from build123d import *

# Parameters (mm, degrees)
CROQUIS1_R               = 18.5
SALIENTE_EXTRUIR1_DEPTH  = 5
CROQUIS2_R               = 0.75
CORTAR_EXTRUIR1_DEPTH    = 5
CROQUIS3_R               = 17.5
CROQUIS3_R_2             = 2.5
CORTAR_EXTRUIR4_DEPTH    = 5
SALIENTE_EXTRUIR11_START = -5
CROQUIS6_W               = 17.427059278
CROQUIS6_H               = 4
SALIENTE_EXTRUIR11_DEPTH = 5
CROQUIS8_W               = 17.261171747
CROQUIS8_H               = 4
SALIENTE_EXTRUIR12_DEPTH = 5


with BuildPart() as part:
    # Croquis1 → Saliente-Extruir1 (new body)
    with BuildSketch(Plane.XY):
        with Locations((-21.322301086, 7.958835432)):
            Circle(CROQUIS1_R)
    extrude(amount=SALIENTE_EXTRUIR1_DEPTH)

    # Croquis2 → Cortar-Extruir1 (cut)
    with BuildSketch(Plane(origin=(0, 0, 0), x_dir=(-1, 0, 0), z_dir=(0, 0, -1))):
        with Locations((21.322301086, 7.958835432)):
            Circle(CROQUIS2_R)
    extrude(amount=-CORTAR_EXTRUIR1_DEPTH, mode=Mode.SUBTRACT)

    # Croquis3 → Cortar-Extruir4 (cut)
    with BuildSketch(Plane.XY.offset(5)):
        with Locations((-21.322301086, 7.958835432)):
            Circle(CROQUIS3_R)
        with Locations((-21.322301086, 7.958835432)):
            Circle(CROQUIS3_R_2, mode=Mode.SUBTRACT)
    extrude(amount=-CORTAR_EXTRUIR4_DEPTH, mode=Mode.SUBTRACT)


with BuildPart() as cortar_extruir4_piece_1:
    # of the separate pieces the step leaves, piece 1, a body of its own (cortar_extruir4_pieces)
    add(part.part.solids().sort_by_distance((-2.822301086, 7.958835432, 0))[0])



with BuildPart() as cortar_extruir4_piece_2:
    # of the separate pieces the step leaves, piece 2, a body of its own (cortar_extruir4_pieces)
    add(part.part.solids().sort_by_distance((-18.822301086, 7.958835432, 0))[0])


with BuildPart() as cortar_extruir4_piece_1_1:
    add(cortar_extruir4_piece_1.part)

    add(cortar_extruir4_piece_2.part)  # Saliente-Extruir11 merges Cortar-Extruir4 piece 2
    # Croquis6 → Saliente-Extruir11 (add)
    with BuildSketch(Plane.XY.offset(5).offset(SALIENTE_EXTRUIR11_START)):
        with Locations((-31.000345605, 7.958835432)):
            Rectangle(CROQUIS6_W, CROQUIS6_H)
    extrude(amount=SALIENTE_EXTRUIR11_DEPTH)

    # Croquis8 → Saliente-Extruir12 (add)
    with BuildSketch(Plane.XY.offset(5)):
        with Locations((-11.561312802, 7.958835432)):
            Rectangle(CROQUIS8_W, CROQUIS8_H)
    extrude(amount=-SALIENTE_EXTRUIR12_DEPTH)


solid = cortar_extruir4_piece_1_1.part
Here's how the part is built. I have some questions about the finished solid (model axes, mm). A direction names the side the tool comes from. Round coordinates to 2 decimals unless told otherwise and drop trailing zeros. Order: outer loops, then holes, each group sorted by start corner. A loop starts at its lowest first (then second) coordinate and runs counter-clockwise, first axis right, second up. Notation, with made-up numbers: M -4,35 L 17,35 A33 cw 17,68 Z; hole C 37,45.25 d7. An arc over 180 degrees is marked long. One line per question, with ' | ' between items.
1) I'm going to push flat-ended pins straight in: pin 1 Ø2.5 at (x, z) = (-27, 2.5) entering from -Y; pin 2 Ø1.5 at (x, z) = (-12, 3) entering from -Y; pin 3 Ø2.5 at (x, z) = (-14, 3) entering from +Y. Where does each tip first touch, or does it pass through?
Checked values:
pin 1: stops at y = -10 | pin 2: stops at y = -8.44 | pin 3: stops at y = 25.43
2) I need wall thicknesses on line 1 (Y direction, x = -31, z = 0.55); line 2 (Y direction, x = -13.5, z = 1.9); line 3 (X direction, y = 16.5, z = 2.1). Which ranges of each line are inside material? Lowest first, please.
Checked values:
line 1: y = -7.81 to -6.62, 5.96 to 9.96, 22.54 to 23.73 | line 2: y = -8.81 to -7.7, 5.96 to 9.96, 23.61 to 24.72 | line 3: x = -37.73 to -36.6, -6.05 to -4.91
3) Imagine slicing it at A-A, the plane y = 17.5. Write out the boundary of the cut face in (x, z), plus the area to 3 significant figures.
Checked values:
outline: M -37.17,0 L -35.99,0 L -35.99,5 L -37.17,5 Z; M -6.65,0 L -5.47,0 L -5.47,5 L -6.65,5 Z | area: 11.8 mm²
4) Imagine slicing it at B-B, the plane x = -8. Write out the boundary of the cut face in (y, z), plus the area to 3 significant figures.
Checked values:
outline: M -4.88,0 L -3.39,0 L -3.39,5 L -4.88,5 Z; M 5.96,0 L 9.96,0 L 9.96,5 L 5.96,5 Z; M 19.31,0 L 20.79,0 L 20.79,5 L 19.31,5 Z | area: 34.9 mm²
5) Imagine slicing it at D-D, the plane y = 1. Write out the boundary of the cut face in (x, z), plus the area to 3 significant figures.
Checked values:
outline: M -38.46,0 L -37.38,0 L -37.38,5 L -38.46,5 Z; M -5.27,0 L -4.18,0 L -4.18,5 L -5.27,5 Z | area: 10.8 mm²
6) On a 3-axis mill with a long thin cutter (end or side, diameter ignored), from which of +Z, -Z, +X, -X, +Y, -Y can I reach the whole of each face in a straight line? I mean faces 1 (the cylindrical face through (-21.34, 5.46, 2.54)), 2 (the flat face through (-21, 9, 5)). Say none if no direction works.
Checked values:
face 1: +Z, -Z | face 2: +Z, +X, -X, +Y, -Y
7) Imagine slicing it at C-C, the plane z = 2.35. Write out the boundary of the cut face in (x, y).
Checked values:
outline: C -21.32,7.96 d37; hole M -38.71,5.96 A17.5 ccw -3.94,5.96 L -19.82,5.96 A2.5 cw -22.82,5.96 Z; hole M -38.71,9.96 L -22.82,9.96 A2.5 cw -19.82,9.96 L -3.94,9.96 A17.5 ccw Z; hole C -21.32,7.96 d1.5
